```python
from build123d import *

# Parameters (mm, degrees)
EXTRUDE_1_DEPTH        = 6
CUT_EXTRUDE_1_DEPTH    = 6
CUT_EXTRUDE_2_DEPTH    = 6
PATTERN_LINEAR_1_COUNT = 2
PATTERN_LINEAR_1_PITCH = 90
FILLET_1_R             = 3


with BuildPart() as part:
    # 草图1 → 凸台-拉伸1 (new body)
    with BuildSketch(Plane.XY):
        Polygon((120, 40), (140, 34), (170, 34), (170, 6), (140, 6), (120, 0), (0, 0), (0, 40), align=None)
    extrude(amount=EXTRUDE_1_DEPTH)

    # 草图2 → 切除-拉伸1 (cut)
    with BuildSketch(Plane.XY.offset(6)):
        with BuildLine():
            Line((10, 23.25), (26, 23.25))
            ThreePointArc((26, 23.25), (29.25, 20), (26, 16.75))
            Line((26, 16.75), (10, 16.75))
            ThreePointArc((10, 16.75), (6.75, 20), (10, 23.25))
        make_face()
    cut_extrude_1 = extrude(amount=-CUT_EXTRUDE_1_DEPTH, mode=Mode.SUBTRACT)

    # 草图3 → 切除-拉伸2 (cut)
    with BuildSketch(Plane.XY.offset(6)):
        with BuildLine():
            Line((140, 23.1), (162, 23.1))
            ThreePointArc((162, 23.1), (165.1, 20), (162, 16.9))
            Line((162, 16.9), (140, 16.9))
            ThreePointArc((140, 16.9), (136.9, 20), (140, 23.1))
        make_face()
    extrude(amount=-CUT_EXTRUDE_2_DEPTH, mode=Mode.SUBTRACT)

    # 阵列(线性)1: 切除-拉伸1 ×2
    with Locations(*[(i * PATTERN_LINEAR_1_PITCH, 0, 0) for i in range(1, PATTERN_LINEAR_1_COUNT)]):
        add(cut_extrude_1, mode=Mode.SUBTRACT)

    # 圆角1
    fillet_1_edges = [part.edges().sort_by_distance(p)[0] for p in [
        (0, 40, 3),
        (170, 34, 3),
        (170, 6, 3),
        (0, 0, 3),
    ]]
    fillet(fillet_1_edges, radius=FILLET_1_R)


solid = part.part
```
Design review of the part built by this model. Coordinates are the model's own, in mm. A direction names the side the tool comes from. Round coordinates to 2 decimals unless told otherwise and drop trailing zeros. Write each loop counter-clockwise with the first axis right and the second up, starting at its lowest first coordinate (ties: lowest second). Pieces come first, ordered by that corner, then holes. Notation, with made-up numbers: (37, 12) -> (91, 12) arc R24 ccw to (91, 34) -> close; hole circle Ø5 at (47.5, 30.5). An arc over 180 degrees is marked (long way). Answer in a Markdown table with one row per item.
Q1. Take a section at C-C, the plane x = 108.5. State the section outline as (y, z) points, then the cut area to 3 significant figures.
The answers:
| item | result |
|---|---|
| outline | (0, 0) -> (16.75, 0) -> (16.75, 6) -> (0, 6) -> close; (23.25, 0) -> (40, 0) -> (40, 6) -> (23.25, 6) -> close |
| area | 201 mm² |
Q2. Draft analysis for pull direction Y (two halves, no side actions). For faces 4 (the face through (0, 20, 3)), 5 (the face through (153, 34, 3)), 6 (the face through (29.25, 20.07, 3.04)), state which applies: +Y half, -Y half, draft (parallel to the pull), parting line (faces both ways), or undercut.
The answers:
| item | result |
|---|---|
| face 4 | draft |
| face 5 | +Y half |
| face 6 | undercut |
Q3. Take a section at B-B, the plane y = 20. State the section outline as (x, z) points, then the cut area to 3 significant figures.
The answers:
| item | result |
|---|---|
| outline | (0, 0) -> (6.75, 0) -> (6.75, 6) -> (0, 6) -> close; (29.25, 0) -> (96.75, 0) -> (96.75, 6) -> (29.25, 6) -> close; (119.25, 0) -> (136.9, 0) -> (136.9, 6) -> (119.25, 6) -> close; (165.1, 0) -> (170, 0) -> (170, 6) -> (165.1, 6) -> close |
| area | 581 mm² |
Q4. Take a section at A-A, the plane z = 1.1. State the section outline as (x, y) points, then the cut area to 3 significant figures.
The answers:
| item | result |
|---|---|
| outline | (0, 3) arc R3 ccw to (3, 0) -> (120, 0) -> (140, 6) -> (167, 6) arc R3 ccw to (170, 9) -> (170, 31) arc R3 ccw to (167, 34) -> (140, 34) -> (120, 40) -> (3, 40) arc R3 ccw to (0, 37) -> close; hole (10, 16.75) -> (26, 16.75) arc R3.25 ccw to (26, 23.25) -> (10, 23.25) arc R3.25 ccw to start; hole (100, 16.75) -> (116, 16.75) arc R3.25 ccw to (116, 23.25) -> (100, 23.25) arc R3.25 ccw to start; hole (140, 16.9) -> (162, 16.9) arc R3.1 ccw to (162, 23.1) -> (140, 23.1) arc R3.1 ccw to start |
| area | 5,870 mm² |
Q5. For faces 1 (the face through (154, 6, 3)), 2 (the face through (96.75, 19.93, 3.04)), 3 (the face through (62, 0, 3)), list the 3-axis set-ups (+Z, -Z, +X, -X, +Y, -Y) from which the entire face can be reached by the end or side of a thin tool; tool diameter is ignored.
The answers:
| item | result |
|---|---|
| face 1 | +Z, -Z, +X, -Y |
| face 2 | +Z, -Z |
| face 3 | +Z, -Z, +X, -X, -Y |
Q6. To check wall thickness, follow L1, parallel to Y at x = 144.5, z = 2.65; L2, parallel to X at y = 18.5, z = 5.35; L3, parallel to Y at x = 12, z = 0.9. State the ranges of each line that lie inside material, in increasing order. Write a range as [from, to].
The answers:
| item | result |
|---|---|
| L1 | [6, 16.9], [23.1, 34] |
| L2 | [0, 7.12], [28.88, 97.12], [118.88, 137.29], [164.71, 170] |
| L3 | [0, 16.75], [23.25, 40] |
Q7. Clearance check with flat-ended pins moving along their axes: pin 1 Ø3 at (x, z) = (146, 3.5) entering from -Y; pin 2 Ø3 at (x, z) = (152, 3.5) entering from +Y. State where each tip first meets the part, or that it passes through.
The answers:
| item | result |
|---|---|
| pin 1 | y = 6 |
| pin 2 | y = 34 |
